from build123d import *

# Parameters (mm, degrees)
SKETCH_1_24X19_W         = 19
SKETCH_1_24X19_H         = 24
EXTRUDE_1_33_DEPTH       = 33
CUT_EXTRUDE_2_REACH      = 38.377
CUT_EXTRUDE_4_2_DEPTH    = 1.9
CUT_EXTRUDE_6_3_REACH    = 29.71
SKETCH_7_5_W             = 24
SKETCH_7_5_H             = 19
EXTRUDE_7_DEPTH          = 5
CUT_EXTRUDE_10_4_REACH   = 41.925
SKETCH_11_W              = 8.5
SKETCH_11_H              = 3.1
CUT_EXTRUDE_11_5_DEPTH   = 4.9
SKETCH_11D1_W            = 6
SKETCH_11D1_H            = 3.1
CUT_EXTRUDE_11D1_6_DEPTH = 10
CUT_EXTRUDE_12_9_REACH   = 31.655
CUT_EXTRUDE_11_DEPTH     = 3.5
SKETCH_5902_W            = 53.98
SKETCH_5902_H            = 19
CUT_EXTRUDE_12_DEPTH     = 1
CUT_EXTRUDE_13_DEPTH     = 40.102429623
CUT_EXTRUDE_15_REACH     = 33.036
SKETCH_5020_R            = 3.5
EXTRUDE_2_DEPTH          = 0.4
SKETCH_7444_W            = 0.8
SKETCH_7444_H            = 3.1
EXTRUDE_3_DEPTH          = 19
CUT_EXTRUDE_16_DEPTH     = 32.036269144


with BuildPart() as part:
    # 1底部方形_24x19 → 1凸台-拉伸_高33 (new body)
    with BuildSketch(Plane(origin=(0, 0, 0), x_dir=(0, 1, 0), z_dir=(0, 0, 1))):
        Rectangle(SKETCH_1_24X19_W, SKETCH_1_24X19_H)
    extrude(amount=EXTRUDE_1_33_DEPTH)

    # 2吸嘴停靠渐变槽 → 2切除-拉伸 (cut, up to next)
    with BuildSketch(Plane.XY.offset(33), mode=Mode.PRIVATE) as cut_extrude_2_sk1:
        with BuildLine():
            Line((12, -5.1), (12, 5.1))
            Line((12, 5.1), (-1.9, 5.1))
            add(Edge.make_bspline(
                [(-5.213938048, 3.830222216), (-3.829124073, 5.093205317), (-1.9, 5.1)],
                knots=[0, 0, 0, 1, 1, 1], degree=2))
            ThreePointArc((-5.213938048, 3.830222216), (-7, 0), (-5.213938048, -3.830222216))
            add(Edge.make_bspline(
                [(-5.213938048, -3.830222216), (-3.829124073, -5.093205317), (-1.9, -5.1)],
                knots=[0, 0, 0, 1, 1, 1], degree=2))
            Line((-1.9, -5.1), (12, -5.1))
        make_face()
    cut_extrude_2_tool1 = extrude(cut_extrude_2_sk1.sketch, amount=-CUT_EXTRUDE_2_REACH, mode=Mode.PRIVATE) & part.part
    add(cut_extrude_2_tool1.solids().sort_by_distance((3.017719, 0, 33))[0], mode=Mode.SUBTRACT)

    # 4反光板停靠槽 → 4切除-拉伸2 (cut)
    with BuildSketch(Plane.XY.offset(25)):
        with BuildLine():
            Line((-0.7, 8.4), (12, 8.4))
            Line((12, 8.4), (12, -8.4))
            Line((12, -8.4), (-0.7, -8.4))
            ThreePointArc((-0.7, -8.4), (-10.5, 0), (-0.7, 8.4))
        make_face()
    extrude(amount=-CUT_EXTRUDE_4_2_DEPTH, mode=Mode.SUBTRACT)

    # 6反光板小圆柱 → 6切除-拉伸3 (cut, up to next)
    with BuildSketch(Plane.XY.offset(23.1), mode=Mode.PRIVATE) as cut_extrude_6_3_sk1:
        with BuildLine():
            Line((-2.1, -6.3), (12, -6.3))
            Line((12, -6.3), (12, 6.3))
            Line((12, 6.3), (-2.1, 6.3))
            ThreePointArc((-2.1, 6.3), (-8.4, 0), (-2.1, -6.3))
        make_face()
    cut_extrude_6_3_tool1 = extrude(cut_extrude_6_3_sk1.sketch, amount=-CUT_EXTRUDE_6_3_REACH, mode=Mode.PRIVATE) & part.part
    add(cut_extrude_6_3_tool1.solids().sort_by_distance((2.424095, 0, 23.1))[0], mode=Mode.SUBTRACT)

    # 7草图5 → 7凸台-拉伸_底板厚度 (add)
    with BuildSketch(Plane(origin=(0, 0, 0), x_dir=(1, 0, 0), z_dir=(0, 0, -1))):
        Rectangle(SKETCH_7_5_W, SKETCH_7_5_H)
    extrude(amount=-EXTRUDE_7_DEPTH)

    # 10切除-拉伸4: up to this face of the body (flat: up to its plane)
    cut_extrude_10_4_end = Plane(part.part.faces().sort_by_distance((0, -9.5, 16.5))[0])
    # Sketch 10 → 10切除-拉伸4 (cut, up to the picked face)
    with BuildSketch(Plane(origin=(0, 9.5, 0), x_dir=(-1, 0, 0), z_dir=(0, 1, 0)), mode=Mode.PRIVATE) as cut_extrude_10_4_sk1:
        Polygon((-12, 31.162738066), (-12, 33), (9, 33), align=None)
    cut_extrude_10_4_tool1 = split(extrude(cut_extrude_10_4_sk1.sketch, amount=-CUT_EXTRUDE_10_4_REACH, mode=Mode.PRIVATE), bisect_by=cut_extrude_10_4_end, keep=Keep.BOTH, mode=Mode.PRIVATE)
    add(cut_extrude_10_4_tool1.solids().sort_by(Axis((5, 9.5, 32.387579), (0, -1, 0)))[0], mode=Mode.SUBTRACT)

    # Sketch 11 → 11切除-拉伸5 (cut)
    with BuildSketch(Plane(origin=(-12, 0, 0), x_dir=(0, -1, 0), z_dir=(-1, 0, 0))):
        with Locations((-5.25, 26.95)):
            Rectangle(SKETCH_11_W, SKETCH_11_H)
        with Locations((5.25, 26.95)):
            Rectangle(SKETCH_11_W, SKETCH_11_H)
    extrude(amount=-CUT_EXTRUDE_11_5_DEPTH, mode=Mode.SUBTRACT)

    # 11d1_磁铁开窗 → 11d1切除-拉伸6 (cut)
    with BuildSketch(Plane(origin=(-12, 0, 0), x_dir=(0, -1, 0), z_dir=(-1, 0, 0))):
        with Locations((0, 26.95)):
            Rectangle(SKETCH_11D1_W, SKETCH_11D1_H)
    extrude(amount=-CUT_EXTRUDE_11D1_6_DEPTH, mode=Mode.SUBTRACT)

    # 12切除薄壁 → 12切除-拉伸9 (cut, up to next)
    with BuildSketch(Plane.XY.offset(25.4), mode=Mode.PRIVATE) as cut_extrude_12_9_sk1:
        with BuildLine():
            Line((-0.7, 8.4), (-0.7, -8.4))
            ThreePointArc((-0.7, -8.4), (-10.5, 0), (-0.7, 8.4))
        make_face()
    cut_extrude_12_9_tool1 = extrude(cut_extrude_12_9_sk1.sketch, amount=-CUT_EXTRUDE_12_9_REACH, mode=Mode.PRIVATE) & part.part
    add(cut_extrude_12_9_tool1.solids().sort_by_distance((-4.916056, 0, 25.4))[0], mode=Mode.SUBTRACT)

    # Sketch 5392 → 切除-拉伸11 (cut)
    with BuildSketch(Plane.XY.offset(33)):
        with BuildLine():
            Line((-2.099999748, 6.5), (12, 6.5))
            Line((12, 6.5), (12, -6.5))
            Line((12, -6.5), (-2.099999748, -6.5))
            ThreePointArc((-2.099999748, -6.5), (-8.6, 0), (-2.099999748, 6.5))
        make_face()
    extrude(amount=-CUT_EXTRUDE_11_DEPTH, mode=Mode.SUBTRACT)

    # Sketch 5902 → 切除-拉伸12 (cut)
    with BuildSketch(Plane.XY.offset(33)):
        with Locations((14.99, 0)):
            Rectangle(SKETCH_5902_W, SKETCH_5902_H)
    extrude(amount=-CUT_EXTRUDE_12_DEPTH, mode=Mode.SUBTRACT)

    # Sketch 6207 → 切除-拉伸13 (cut, through all)
    with BuildSketch(Plane.XZ.offset(9.5)):
        Polygon((2.430052303, 32), (12, 31.162738066), (12, 28.826114347), (-6, 32), align=None)
    extrude(amount=-CUT_EXTRUDE_13_DEPTH, mode=Mode.SUBTRACT)

    # Sketch 5020 → 切除-拉伸15 (cut, up to next)
    with BuildSketch(Plane.XY.offset(5), mode=Mode.PRIVATE) as cut_extrude_15_sk1:
        with Locations((2, 0)):
            Circle(SKETCH_5020_R)
    cut_extrude_15_tool1 = extrude(cut_extrude_15_sk1.sketch, amount=-CUT_EXTRUDE_15_REACH, mode=Mode.PRIVATE) & part.part
    add(cut_extrude_15_tool1.solids().sort_by_distance((2, 0, 5))[0], mode=Mode.SUBTRACT)

    # Sketch 6982 → 凸台-拉伸2 (add)
    with BuildSketch(Plane(origin=(0, 0, 25.4), x_dir=(1, 0, 0), z_dir=(0, 0, -1))):
        with BuildLine():
            Line((-7.1, -3), (-7.1, -6.8))
            ThreePointArc((-7.1, -6.8), (-4.061552813, -8.246211251), (-0.7, -8.4))
            Line((-0.7, -8.4), (-0.7, -5.1))
            Line((-0.7, -5.1), (-1.9, -5.1))
            add(Edge.make_bspline(
                [(-1.9, -5.1), (-3.829124073, -5.093205317), (-5.213938048, -3.830222216)],
                knots=[0, 0, 0, 1, 1, 1], degree=2))
            ThreePointArc((-5.213938048, -3.830222216), (-5.630777158, -3.437652866), (-6, -3))
            Line((-6, -3), (-7.1, -3))
        make_face()
        with BuildLine():
            Line((-7.1, 3), (-6, 3))
            ThreePointArc((-6, 3), (-5.630777158, 3.437652866), (-5.213938048, 3.830222216))
            add(Edge.make_bspline(
                [(-5.213938048, 3.830222216), (-3.829124073, 5.093205317), (-1.9, 5.1)],
                knots=[0, 0, 0, 1, 1, 1], degree=2))
            Line((-1.9, 5.1), (-0.7, 5.1))
            Line((-0.7, 5.1), (-0.7, 8.4))
            ThreePointArc((-0.7, 8.4), (-4.061552813, 8.246211251), (-7.1, 6.8))
            Line((-7.1, 6.8), (-7.1, 3))
        make_face()
    extrude(amount=EXTRUDE_2_DEPTH)

    # Sketch 7444 → 凸台-拉伸3 (add)
    with BuildSketch(Plane.XZ.offset(9.5)):
        with Locations((-11.6, 26.95)):
            Rectangle(SKETCH_7444_W, SKETCH_7444_H)
    extrude(amount=-EXTRUDE_3_DEPTH)

    # 草图13 → 切除-拉伸16 (cut, through all)
    with BuildSketch(Plane.XY.offset(5)):
        with BuildLine():
            Line((-2.1, -6.3), (12, -6.3))
            Line((12, -6.3), (12, 6.3))
            Line((12, 6.3), (-2.1, 6.3))
            ThreePointArc((-2.1, 6.3), (-8.4, 0), (-2.1, -6.3))
        make_face()
    extrude(amount=-CUT_EXTRUDE_16_DEPTH, mode=Mode.SUBTRACT)


solid = part.part
Geometry check sheet. Reference: the model listing, model coordinates, mm. A direction names the side the tool comes from. Round coordinates to 2 decimals unless told otherwise and drop trailing zeros. Order: outer loops, then holes, each group sorted by start corner. A loop starts at its lowest first (then second) coordinate and runs counter-clockwise, first axis right, second up. Notation, with made-up numbers: M -29.5,-17 L 4.5,-17 A15 cw 4.5,-7 Z; hole C 29,4 d1. An arc over 180 degrees is marked long. Answer in a Markdown table with one row per item. Add a question column.
Item 1: Depth check by flat-ended pin: pin 1 Ø3 at (x, y) = (5.5, -4.5) entering from -Z; pin 2 Ø8.5 at (x, y) = (5.5, -2) entering from +Z; pin 3 Ø0.9 at (x, z) = (3, 30.5) entering from -Y; pin 4 Ø3.5 at (y, z) = (-3, 26.5) entering from +X. Enter the tip coordinate at first touch or a pass-through.
Item 2: Set-up check for faces 1 (the face through (-6.6, -3, 26.8)), 2 (the face through (-0.8, 5.3, 29.5)), 3 (the face through (5, 5.1, 27)): record each of +Z, -Z, +X, -X, +Y, -Y from which the full face is reachable in a straight line by a thin tool's end or side.
Item 3: Sectioned sample at B-B, the plane z = 2. Enter the section's corners in (x, y).
Item 4: Sectioned sample at A-A, the plane x = -9.5. Enter the section's corners in (y, z), plus the area to 3 significant figures.
Item 5: Draft check along Z on faces 4 (the face through (-8.2, -2.2, 0)), 5 (the face through (0, 9.5, 16)), 6 (the face through (-7.1, 6, 27)), 7 (the face through (-11, 0, 25.4)). Enter one of: released by +Z, released by -Z, zero draft, split by the parting line, or undercut.
Item 6: Sectioned sample at D-D, the plane x = 0. Enter the section's corners in (y, z), plus the area to 3 significant figures.
Item 7: Material ranges on L1, parallel to Y at x = -0.25, z = 17.5; L2, parallel to Y at x = -2, z = 23.95; L3, parallel to Z at x = -10.25, y = -6.5, recorded low to high. Write a range as [from, to].
Item 8: Sectioned sample at C-C, the plane y = 0. Enter the section's corners in (x, z).
Filled in:
| question | item | result |
|---|---|---|
| 1 | pin 1 | stops at z = 25 |
| 1 | pin 2 | stops at z = 29.5 |
| 1 | pin 3 | stops at y = -9.5 |
| 1 | pin 4 | stops at x = -3.77 |
| 2 | face 1 | -Z, +X |
| 2 | face 2 | +Z, +X |
| 2 | face 3 | +Z, -Z, +X |
| 3 | outline | M -12,-9.5 L 12,-9.5 L 12,-6.3 L -2.1,-6.3 A6.3 cw -2.1,6.3 L 12,6.3 L 12,9.5 L -12,9.5 Z |
| 4 | outline | M -9.5,0 L 9.5,0 L 9.5,25.4 L 4,25.4 L 4,23.1 L -4,23.1 L -4,25.4 L -9.5,25.4 Z; M -9.5,28.5 L 9.5,28.5 L 9.5,32 L -9.5,32 Z |
| 4 | area | 531 mm² |
| 5 | face 4 | released by -Z |
| 5 | face 5 | zero draft |
| 5 | face 6 | undercut |
| 5 | face 7 | undercut |
| 6 | outline | M -9.5,0 L -6.3,0 L -6.3,23.1 L -8.4,23.1 L -8.4,25 L -5.1,25 L -5.1,29.5 L -6.5,29.5 L -6.5,30.94 L -9.5,30.94 Z; M 5.1,25 L 8.4,25 L 8.4,23.1 L 6.3,23.1 L 6.3,0 L 9.5,0 L 9.5,30.94 L 6.5,30.94 L 6.5,29.5 L 5.1,29.5 Z |
| 6 | area | 200 mm² |
| 7 | L1 | y = [-9.5, -6.3], [6.3, 9.5] |
| 7 | L2 | y = [-9.5, -8.5], [8.5, 9.5] |
| 7 | L3 | z = [0, 25.4], [28.5, 32] |
| 8 | outline | M -12,0 L -8.4,0 L -8.4,23.1 L -10.5,23.1 L -10.5,25.4 L -11.2,25.4 L -11.2,28.5 L -7,28.5 L -7,29.5 L -8.6,29.5 L -8.6,32 L -12,32 Z |
